from build123d import *

# Parameters (mm, degrees)
F1_DEPTH = 5
F3_DEPTH = 3
F4_R     = 20
F5_R     = 21
F7_DEPTH = 2


with BuildPart() as f1:
    # F0 (on Right) → F1 (new body)
    with BuildSketch(Plane.YZ):
        Polygon((-2.6435090923, -26.501225133), (5.3746857459, -26.501225133), (5.3746857459, -16.4436940104), (-55.1649013234, -3.4599144195), (-14.2791476101, -26.501225133), (-22.9189545176, -44.7233500122), (-14.2791476101, -51.0418266058), align=None)
        Polygon((-55.1649013234, -3.4599144195), (5.3746857459, -16.4436940104), (5.3746857459, 12.498774867), (-52.7289716819, 22.7440173494), (-70.3398138285, -14.3988225609), (-62.8945189948, -19.4552624983), align=None)
    extrude(amount=F1_DEPTH)

    # F2 (on face) → F3 (join)
    with BuildSketch(Plane.YZ.offset(5)):
        Polygon((5.3746857459, 12.498774867), (-52.7289716819, 22.7440173494), (-70.3398138285, -14.3988225609), (-68.6655286126, -15.5359061582), (-51.5614379211, 20.5381496464), (5.3746857459, 10.498774867), align=None)
    extrude(amount=F3_DEPTH)

    # F4
    f4_edges = [f1.edges().sort_by_distance(p)[0] for p in [
        (6.5, -51.561438, 20.53815),
    ]]
    fillet(f4_edges, radius=F4_R)

    # F5
    f5_edges = [f1.edges().sort_by_distance(p)[0] for p in [
        (4, -52.728972, 22.744017),
    ]]
    fillet(f5_edges, radius=F5_R)

    # F6 (on face) → F7 (cut)
    with BuildSketch(Plane(origin=(0, 0, 0), x_dir=(0, -1, 0), z_dir=(-1, 0, 0))):
        Polygon((2.6435090923, 13.9125989535), (-5.3746857459, 12.498774867), (-5.3746857459, -26.501225133), (2.6435090923, -26.501225133), align=None)
    extrude(amount=-F7_DEPTH, mode=Mode.SUBTRACT)


solid = f1.part
Source: CAD feature listing. Evaluate the final solid. Frame: model axes, mm. A direction names the side the tool comes from. Round coordinates to 2 decimals unless told otherwise and drop trailing zeros. Loops run counter-clockwise (first coordinate to the right, second up) from the corner with the lowest first, then second, coordinate; pieces in that order, holes last.
Q1. Section D-D, the plane z = 0.5. Return loops of the section in (x, y), plus the area to 3 significant figures.
Q2. Access query for faces 4 (the face through (2.46, -35.01, -14.82)), 5 (the face through (6.521, -49.037, 16.047)), 6 (the face through (2, 1, -6)). Directions: +Z, -Z, +X, -X, +Y, -Y. A direction counts if a zero-diameter tool reaches every point of the face in a straight line with its end or side. Return the directions, or none.
Q3. Section B-B, the plane x = 1. Return loops of the section in (y, z) (1 decimal).
Q4. First-contact query: P1, Ø0.6, axis at x = 1, z = -4.5, coming from the +Y side; P2, Ø10, axis at y = -28.5, z = -38, coming from the -X side; P3, Ø8, axis at y = -20, z = -27, coming from the -X side; P4, Ø21, axis at y = -38.5, z = -0.5, coming from the +X side. Flat tips, straight axial feed; report the tip coordinate or a pass-through.
Q5. Section A-A, the plane z = -9. Return loops of the section in (x, y), plus the area to 3 significant figures.
Q6. Section C-C, the plane y = -21.5. Return loops of the section in (x, z), plus the area to 3 significant figures.
Q7. Ray query, line 1 (X direction, y = -2, z = 3); line 2 (Y direction, x = 4, z = -13.5); line 3 (Y direction, x = 1.75, z = -6). Return the intervals inside material, ascending.
Q8. Mould query, pull axis Y, two halves, no side actions, for faces 1 (the face through (0, -29, -7)), 2 (the face through (2.5, -59.1, -11.6)), 3 (the face through (2.465, -18.539, -35.485)). Classes: pulls with the +Y half, pulls with the -Y half, needs draft (parallel to the pull), parting line crosses it, or undercut.
Solutions:
1. outline: (0, -63.28) - (8, -63.28) - (8, -61.06) - (5, -61.06) - (5, 5.37) - (2, 5.37) - (2, -2.64) - (0, -2.64) - close
1. area: 334 mm2
2. face 4: +X, -X
2. face 5: -Z, +X
2. face 6: +Z, -Z, -X, +Y
3. outline: (-70.3, -14.4) - (-62.9, -19.5) - (-55.2, -3.5) - (-14.3, -26.5) - (-22.9, -44.7) - (-14.3, -51) - (-2.6, -26.5) - (-2.6, 13.9) - (-37, 20) arc R21 ccw to (-59.6, 8.3) - close
4. P1: stops at y = -2.64
4. P2: passes through
4. P3: stops at x = 0
4. P4: stops at x = 5
5. outline: (0, -67.78) - (8, -67.78) - (8, -65.57) - (5, -65.57) - (5, -57.84) - (0, -57.84) - close; (0, -45.33) - (5, -45.33) - (5, 5.37) - (2, 5.37) - (2, -2.64) - (0, -2.64) - close
5. area: 294 mm2
6. outline: (0, -45.76) - (5, -45.76) - (5, -41.73) - (0, -41.73) - close; (0, -22.43) - (5, -22.43) - (5, 15.24) - (8, 15.24) - (8, 17.24) - (0, 17.24) - close
6. area: 224 mm2
7. line 1: x = 2 to 5
7. line 2: y = -69.91 to -60.02, -37.35 to 5.37
7. line 3: y = -66.36 to -56.39, -50.66 to -2.64
8. face 1: needs draft
8. face 2: undercut
8. face 3: pulls with the -Y half
